from build123d import *

# Parameters (mm, degrees)
F0_W     = 108.5735373199
F0_H     = 44.3482641131
F1_DEPTH = 254
F3_DEPTH = 76.2


with BuildPart() as f1:
    # F0 (on Front) → F1 (new body)
    with BuildSketch(Plane.XZ):
        with Locations((2.2877622396, -1.4324570075)):
            Rectangle(F0_W, F0_H)
    extrude(amount=F1_DEPTH)

    # F2 (on face) → F3 (cut)
    with BuildSketch(Plane(origin=(0, 0, -23.606589064), x_dir=(1, 0, 0), z_dir=(0, 0, -1))):
        with BuildLine():
            Line((0, 50.8), (-12.7, 50.8))
            ThreePointArc((-12.7, 50.8), (0, 38.1), (12.7, 50.8))
            Line((12.7, 50.8), (0, 50.8))
        make_face()
        with BuildLine():
            Line((-12.7, 101.6), (-12.7, 50.8))
            ThreePointArc((-12.7, 50.8), (-8.9802561211, 59.7802561211), (0, 63.5))
            Line((0, 63.5), (0, 88.9))
            ThreePointArc((0, 88.9), (-8.9802561211, 92.6197438789), (-12.7, 101.6))
        make_face()
        with BuildLine():
            ThreePointArc((0, 63.5), (-8.9802561211, 59.7802561211), (-12.7, 50.8))
            Line((-12.7, 50.8), (0, 50.8))
            Line((0, 50.8), (0, 63.5))
        make_face()
        with BuildLine():
            Line((0, 50.8), (12.7, 50.8))
            ThreePointArc((12.7, 50.8), (8.9802561211, 59.7802561211), (0, 63.5))
            Line((0, 63.5), (0, 50.8))
        make_face()
        with BuildLine():
            ThreePointArc((0, 63.5), (8.9802561211, 59.7802561211), (12.7, 50.8))
            Line((12.7, 50.8), (12.7, 101.6))
            ThreePointArc((12.7, 101.6), (8.9802561211, 92.6197438789), (0, 88.9))
            Line((0, 88.9), (0, 63.5))
        make_face()
        with BuildLine():
            Line((0, 101.6), (-12.7, 101.6))
            ThreePointArc((-12.7, 101.6), (-8.9802561211, 92.6197438789), (0, 88.9))
            Line((0, 88.9), (0, 101.6))
        make_face()
        with BuildLine():
            ThreePointArc((12.7, 101.6), (0, 114.3), (-12.7, 101.6))
            Line((-12.7, 101.6), (0, 101.6))
            Line((0, 101.6), (12.7, 101.6))
        make_face()
        with BuildLine():
            ThreePointArc((0, 88.9), (8.9802561211, 92.6197438789), (12.7, 101.6))
            Line((12.7, 101.6), (0, 101.6))
            Line((0, 101.6), (0, 88.9))
        make_face()
    extrude(amount=-F3_DEPTH, mode=Mode.SUBTRACT)


solid = f1.part
Geometry check sheet. Reference: the model listing, model coordinates, mm. A direction names the side the tool comes from. Round coordinates to 2 decimals unless told otherwise and drop trailing zeros. Loops run counter-clockwise (first coordinate to the right, second up) from the corner with the lowest first, then second, coordinate; pieces in that order, holes last.
Item 1: Cross-section at B-B on z = 7.5. Record the boundary of the cut face in (x, y).
Item 2: Thickness scan on line 1 (X direction, y = -93, z = -12); line 2 (X direction, y = -103, z = 12); line 3 (Y direction, x = -2, z = 1). Record the ranges inside material, lowest first.
Item 3: Cross-section at A-A on x = 0. Record the boundary of the cut face in (y, z).
Item 4: Access from +Z, -Z, +X, -X, +Y, -Y to the whole of each face (thin tool, end or side, straight path). Record for faces 5 (the cylindrical face through (0.279, -114.297, -1.743)), 6 (the flat face through (2, -125, -23.607)).
Item 5: Mould release check, pull along Y, two halves, no side actions. Record for faces 1 (the flat face through (2, -125, 20.742)), 2 (the flat face through (2, -254, -1)), 3 (the flat face through (-12.7, -77, -2)), 4 (the flat face through (12.7, -76, -2)): pulls with the +Y half, pulls with the -Y half, needs draft (parallel to the pull), parting line crosses it, or undercut.
Answer sheet:
1. outline: (-52, -254) - (56.57, -254) - (56.57, 0) - (-52, 0) - close; hole (-12.7, -101.6) arc R12.7 ccw to (12.7, -101.6) - (12.7, -50.8) arc R12.7 ccw to (-12.7, -50.8) - close
2. line 1: x = -52 to -12.7, 12.7 to 56.57
2. line 2: x = -52 to -12.62, 12.62 to 56.57
2. line 3: y = -254 to -114.14, -38.26 to 0
3. outline: (-254, -23.61) - (-114.3, -23.61) - (-114.3, 20.74) - (-254, 20.74) - close; (-38.1, -23.61) - (0, -23.61) - (0, 20.74) - (-38.1, 20.74) - close
4. face 5: +Z, -Z
4. face 6: -Z, +X, -X, +Y, -Y
5. face 1: needs draft
5. face 2: pulls with the -Y half
5. face 3: undercut
5. face 4: undercut
